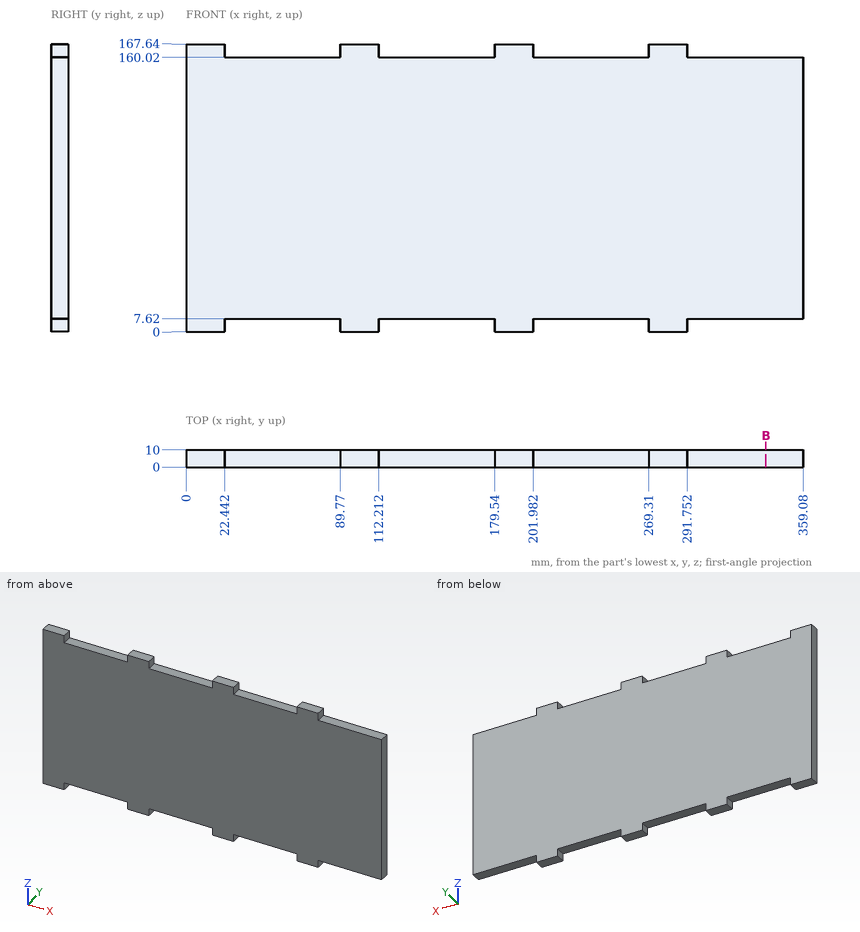
Here's the drawing with two shaded views (mm, measured from the low corner). I have some questions. Round coordinates to 2 decimals unless told otherwise and drop trailing zeros. Order: outer loops, then holes, each group sorted by start corner. A loop starts at its lowest first (then second) coordinate and runs counter-clockwise, first axis right, second up. Notation, with made-up numbers: (84, -2.5) -> (113, -2.5) arc R11 cw to (113, 12.5) -> close; hole circle Ø1 at (-4, 54.5). An arc over 180 degrees is marked (long way). Write each question's results on one line, items separated by ' | '. Start each with the question number.
Item 1: Will these pins go through, and if not, where does the flat tip stop? pin 1 (3 mm diameter, centred on x = 243, y = 2.5, fed in from -Z); pin 2 (2.5 mm diameter, centred on y = 7, z = 5, fed in from +X); pin 3 (5 mm diameter, centred on x = 144, y = 7, fed in from +Z).
Item 2: If we section it at B-B, the plane x = 337.5: Write out the boundary of the cut face in (y, z), then the cut area to 3 significant figures.
Item 3: Please list where this line runs through material, in increasing order: L1, parallel to Z at x = 86.5, y = 6.5.
Results:
1) pin 1: stops at z = 7.62 | pin 2: stops at x = 291.75 | pin 3: stops at z = 160.02
2) outline: (0, 7.62) -> (10, 7.62) -> (10, 160.02) -> (0, 160.02) -> close | area: 1,520 mm2
3) L1: z = 7.62 to 160.02
